Model file for the job. Use its own axes, mm. Round coordinates to 2 decimals unless told otherwise and drop trailing zeros. Order: outer loops, then holes, each group sorted by start corner. A loop starts at its lowest first (then second) coordinate and runs counter-clockwise, first axis right, second up. Notation, with made-up numbers: (-1, 70.5) -> (41, 70.5) arc R19 cw to (41, 100.5) -> close; hole circle Ø7 at (-26.5, 71.25). An arc over 180 degrees is marked (long way). Use CSV: the item, a comma, the result in double quotes.
```python
from build123d import *

# Parameters (mm, degrees)
SKETCH1_R           = 1.5
BOSS_EXTRUDE1_DEPTH = 3
FILLET1_R           = 3
SKETCH2_R           = 29.25
SKETCH2_R_2         = 1.3
CUT_EXTRUDE1_DEPTH  = 3


with BuildPart() as part:
    # Sketch1 → Boss-Extrude1 (new body)
    with BuildSketch(Plane.XY):
        with BuildLine():
            Line((-36, 0), (-36, 48))
            Line((-36, 48), (-71.25, 48))
            Line((-71.25, 48), (-71.25, 100))
            Line((-71.25, 100), (71.25, 100))
            Line((71.25, 100), (71.25, 48))
            Line((71.25, 48), (36, 48))
            Line((36, 48), (36, 0))
            ThreePointArc((36, 0), (0, -36), (-36, 0))
        make_face()
        with Locations((-67.75, 95.75)):
            Circle(SKETCH1_R, mode=Mode.SUBTRACT)
        with Locations((67.75, 95.75)):
            Circle(SKETCH1_R, mode=Mode.SUBTRACT)
        with Locations((67.75, 52.25)):
            Circle(SKETCH1_R, mode=Mode.SUBTRACT)
        with Locations((-67.75, 52.25)):
            Circle(SKETCH1_R, mode=Mode.SUBTRACT)
    extrude(amount=BOSS_EXTRUDE1_DEPTH)

    # Fillet1
    fillet1_edges = [part.edges().sort_by_distance(p)[0] for p in [
        (36, 48, 1.5),
        (-36, 48, 1.5),
    ]]
    fillet(fillet1_edges, radius=FILLET1_R)

    # Sketch2 → Cut-Extrude1 (cut)
    with BuildSketch(Plane.XY.offset(3)):
        Circle(SKETCH2_R)
        with Locations((12.724224126, 30.718994456)):
            Circle(SKETCH2_R_2)
        with Locations((30.718994456, -12.724224126)):
            Circle(SKETCH2_R_2)
        with Locations((-12.724224126, -30.718994456)):
            Circle(SKETCH2_R_2)
        with Locations((-30.718994456, 12.724224126)):
            Circle(SKETCH2_R_2)
    extrude(amount=-CUT_EXTRUDE1_DEPTH, mode=Mode.SUBTRACT)


solid = part.part
```
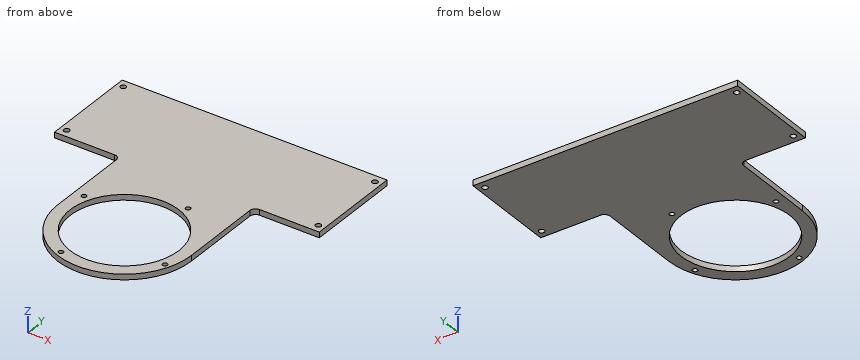
Q1. Pin check, flat tips, straight feed: pin 1 (3 mm diameter, centred on x = -34.5, y = 25, fed in from -Z); pin 2 (1.5 mm diameter, centred on x = 54.5, z = 2, fed in from -Y); pin 3 (1.5 mm diameter, centred on y = 28, z = 2, fed in from -X). Stop position of each tip, or through.
From the geometry:
pin 1,"stops at z = 0"
pin 2,"stops at y = 48"
pin 3,"stops at x = -36"
Q2. Cut at A-A (x = -16.5). Give the cut face in (y, z).
From the geometry:
outline,"(-32, 0) -> (-24.15, 0) -> (-24.15, 3) -> (-32, 3) -> close; (24.15, 0) -> (100, 0) -> (100, 3) -> (24.15, 3) -> close"
Q3. Cut at D-D (x = -62). Give the cut face in (y, z), plus the area to 3 significant figures.
From the geometry:
outline,"(48, 0) -> (100, 0) -> (100, 3) -> (48, 3) -> close"
area,"156 mm²"
Q4. Probe line 1 along X through (y, z) = (95.75, 0.9); line 2 along Y through (x, z) = (67.75, 1.9); line 3 along X through (y, z) = (24, 0.65). List the from-to ranges inside material, lowest first.
From the geometry:
line 1,"x = -71.25 to -69.25, -66.25 to 66.25, 69.25 to 71.25"
line 2,"y = 48 to 50.75, 53.75 to 94.25, 97.25 to 100"
line 3,"x = -36 to -16.72, 16.72 to 36"
Q5. Cut at C-C (z = 0.7). State how many separate pieces and enclosed holes the cut face has, plus the area to 3 significant figures.
From the geometry:
separate pieces,"1"
enclosed holes,"9"
area,"10,200 mm²"
Q6. Cut at B-B (y = -2.5). Give the cut face in (x, z).
From the geometry:
outline,"(-35.91, 0) -> (-29.14, 0) -> (-29.14, 3) -> (-35.91, 3) -> close; (29.14, 0) -> (35.91, 0) -> (35.91, 3) -> (29.14, 3) -> close"
